from build123d import *

# Parameters (mm, degrees)
SKETCH_2_R      = 1.25
SKETCH_2_R_2    = 1.5
EXTRUDE_1_DEPTH = 3


with BuildPart() as part:
    # 草圖2 → 填料-伸長1 (new body)
    with BuildSketch(Plane.XY):
        with BuildLine():
            ThreePointArc((31.771756119, 138.671302862), (28.601861286, 119.774671061), (31.9, 100.9))
            ThreePointArc((31.9, 100.9), (30.360629041, 96.771462466), (25.959440964, 96.561632457))
            ThreePointArc((25.959440964, 96.561632457), (18.105782324, 98.350587579), (10.682096943, 95.22501406))
            ThreePointArc((10.682096943, 95.22501406), (5.16557517, 95.514842117), (5.199291514, 101.038869269))
            ThreePointArc((5.199291514, 101.038869269), (17.826888938, 119.231579997), (24.029658233, 140.490850759))
            ThreePointArc((24.029658233, 140.490850759), (28.365250917, 143.714078762), (32.00050872, 139.717647432))
            ThreePointArc((32.00050872, 139.717647432), (31.917708673, 139.187571923), (31.771756119, 138.671302862))
        make_face()
        with Locations((27.99967116, 140.002243515)):
            Circle(SKETCH_2_R, mode=Mode.SUBTRACT)
        with Locations((8.075611168, 98.259296802)):
            Circle(SKETCH_2_R_2, mode=Mode.SUBTRACT)
        with Locations((27.999548416, 100.002200002)):
            Circle(SKETCH_2_R_2, mode=Mode.SUBTRACT)
    extrude(amount=EXTRUDE_1_DEPTH)


solid = part.part
Verification items for the finished model (mm, model axes). Coordinates: 2 decimals unless noted, no trailing zeros. Order: outer loops, then holes, each group sorted by start corner. A loop starts at its lowest first (then second) coordinate and runs counter-clockwise, first axis right, second up.
1. Sectioned sample at A-A, the plane x = 30.25. Record the cut outline in (y, z).
Results found:
outline: (96.69, 0) - (106.39, 0) - (106.39, 3) - (96.69, 3) - close; (133.55, 0) - (143.03, 0) - (143.03, 3) - (133.55, 3) - close
2. Go/stop test with flat-tipped pins: pin 1 Ø8 at (x, y) = (15.5, 132.5) entering from +Z; pin 2 Ø5 at (x, y) = (28, 100) entering from +Z. Record where each tip stops, or that it passes through.
Results found:
pin 1: passes through
pin 2: stops at z = 3
3. Sectioned sample at B-B, the plane z = 1.45. Record the cut outline in (x, y), and give its area (3 significant figures).
Results found:
outline: (5.2, 101.04) arc R4 ccw to (10.68, 95.23) arc R13.15 cw to (25.96, 96.56) arc R4 ccw to (31.9, 100.9) arc R56.76 cw to (31.77, 138.67) arc R4.45 ccw to (32, 139.72) arc R4.02 ccw to (24.03, 140.49) arc R68.89 cw to start; hole circle Ø3 at (8.08, 98.26); hole circle Ø3 at (28, 100); hole circle Ø2.5 at (28, 140)
area: 613 mm2
4. Scan lines: line 1 (Y direction, x = 28, z = 1.2); line 2 (Y direction, x = 28.5, z = 2.35); line 3 (X direction, y = 101, z = 2.05). Record each from-to range of solid material in increasing order.
Results found:
line 1: y = 96 to 98.5, 101.5 to 138.75, 141.25 to 143.73
line 2: y = 96.03 to 98.59, 101.42 to 138.86, 141.15 to 143.7
line 3: x = 5.16 to 26.88, 29.12 to 31.86
5. Sectioned sample at D-D, the plane x = 8. Record the cut outline in (y, z), and give its area (3 significant figures).
Results found:
outline: (94.26, 0) - (96.76, 0) - (96.76, 3) - (94.26, 3) - close; (99.76, 0) - (104.12, 0) - (104.12, 3) - (99.76, 3) - close
area: 20.6 mm2
6. Release check for a two-part mould opening along X. For faces 1 (the face through (31.92, 139.19, 1.48)), 2 (the face through (30.4, 96.8, 1.5)), 3 (the face through (5.225, 95.453, 1.479)) record: +X half, -X half, draft (parallel to the pull), parting line (faces both ways), or undercut.
Results found:
face 1: +X half
face 2: undercut
face 3: parting line
7. Sectioned sample at C-C, the plane y = 126.5. Record the cut outline in (x, z).
Results found:
outline: (20.8, 0) - (28.98, 0) - (28.98, 3) - (20.8, 3) - close
